CAD build for the part. Positions are in the model's coordinates, mm. Give positions to 0.01 mm unless a question says otherwise; leave off trailing zeros. Write each loop counter-clockwise with the first axis right and the second up, starting at its lowest first coordinate (ties: lowest second). Pieces come first, ordered by that corner, then holes. Notation, with made-up numbers: M 84,60.5 L 118,60.5 A21 cw 118,83.5 Z; hole C 76,-9 d10. An arc over 180 degrees is marked long. One line per question, with ' | ' between items. Start each with the question number.
1. Cut at C-C, the plane x = -8. Write the cut outline in (y, z).
2. Cut at A-A, the plane y = 30.5. Write the cut outline in (x, z) (3 decimals), then the cut area to 3 significant figures.
3. Cut at B-B, the plane z = 5.5. Write the cut outline in (x, y), then the cut area to 3 significant figures.
4. Flat gauge pins, fed straight in: pin 1 (4 mm diameter, centred on x = -8.5, y = 120.5, fed in from -Z); pin 2 (5 mm diameter, centred on x = 0, z = 0, fed in from -Y); pin 3 (5 mm diameter, centred on x = -8, y = 125.5, fed in from -Z); pin 4 (3 mm diameter, centred on x = -12, y = 64, fed in from -Z). Where does each tip first touch, or does it go through?
5. Pull direction Z, two halves, no side cores. Call faces 1 (the face through (1.431, 69.746, -0.593)), 2 (the face through (0, 162.56, 0)), 3 (the face through (-3.441, 80.142, -15.497)): released by +Z, released by -Z, zero draft, split by the parting line, or undercut.
6. Wall check: L1, parallel to Z at x = 0, y = 70 (3 decimals); L2, parallel to Z at x = -8, y = 155; L3, parallel to X at y = 35, z = 14. Give the ranges that are in metal, low to high.
```python
from build123d import *

# Parameters (mm, degrees)
F0_R     = 15.875
F1_DEPTH = 162.56
F2_R     = 1.5494
F3_DEPTH = 142.367
F4_SIZE2 = 1.5494
F4_SIZE  = 0.8945465071


with BuildPart() as f1:
    # F0 (on Front) → F1 (new body)
    with BuildSketch(Plane.XZ):
        Circle(F0_R)
    extrude(amount=-F1_DEPTH)

    # F2 (on Front) → F3 (cut)
    with BuildSketch(Plane.XZ):
        Circle(F2_R)
    extrude(amount=-F3_DEPTH, mode=Mode.SUBTRACT)

    # F4
    f4_edges = [f1.edges().sort_by_distance(p)[0] for p in [
        (-1.5494, 142.367, 0),
    ]]
    f4_side = f1.faces().sort_by_distance((-1.5494, 71.1835, 0))[0]
    chamfer(f4_edges, length=F4_SIZE, length2=F4_SIZE2, reference=f4_side)


solid = f1.part
```
Here are the results:
1) outline: M 0,-13.71 L 162.56,-13.71 L 162.56,13.71 L 0,13.71 Z
2) outline: C 0,0 d31.75; hole C 0,0 d3.099 | area: 784 mm^2
3) outline: M -14.89,0 L 14.89,0 L 14.89,162.56 L -14.89,162.56 Z | area: 4,840 mm^2
4) pin 1: z = -14.48 | pin 2: y = 0 | pin 3: z = -14.89 | pin 4: z = -11.91
5) face 1: undercut | face 2: zero draft | face 3: split by the parting line
6) L1: -15.875 to -1.549, 1.549 to 15.875 | L2: -13.71 to 13.71 | L3: -7.48 to 7.48
